Here's the drawing with two shaded views (mm, measured from the low corner). I have some questions. A direction names the side the tool comes from. Round coordinates to 2 decimals unless told otherwise and drop trailing zeros. Loops run counter-clockwise (first coordinate to the right, second up) from the corner with the lowest first, then second, coordinate; pieces in that order, holes last. Notation, with made-up numbers: (71, 35) -> (125, 35) arc R13 cw to (125, 39) -> close; hole circle Ø10 at (67, -32.75). An arc over 180 degrees is marked (long way). Write item = value, one per line.
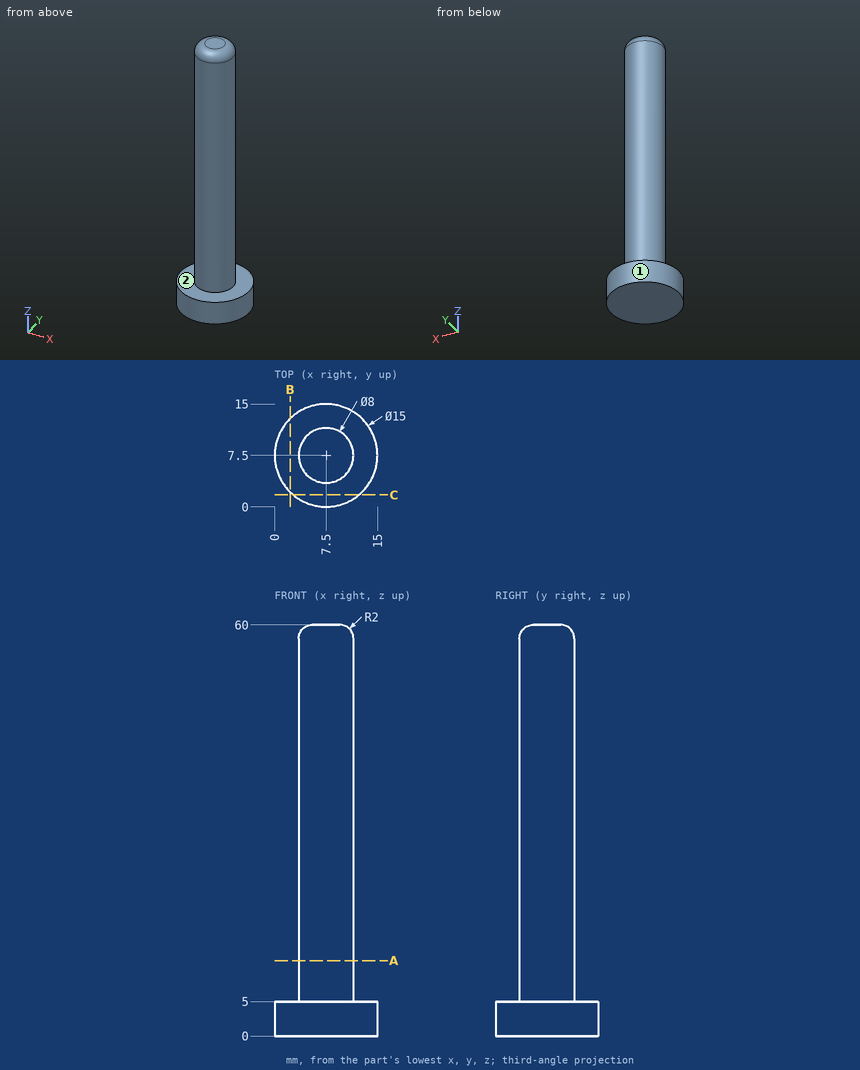
1. Suppose I cut it at A-A, the plane z = 11. List the corners of the cut face in (x, y) for me, and give its area (3 significant figures).
Entries:
outline = circle Ø8 at (7.5, 7.5)
area = 50.3 mm²
2. For the marked faces 1 and 2, which set-ups out of +Z, -Z, +X, -X, +Y, -Y let a thin tool reach every point of the face, with its end or its side?
Entries:
face_1 = +Z, -Z
face_2 = +Z
3. I need wall thicknesses on line 1 (Z direction, x = 11.75, y = 3.5); line 2 (X direction, y = 9.25, z = 34.5); line 3 (Y direction, x = 10.75, z = 42). Which ranges of each line are inside material? Lowest first, please. Write a range as [from, to].
Entries:
line_1 = [0, 5]
line_2 = [3.9, 11.1]
line_3 = [5.17, 9.83]
4. Suppose I cut it at B-B, the plane x = 2.25. List the corners of the cut face in (y, z) for me, and give its area (3 significant figures).
Entries:
outline = (2.14, 0) -> (12.86, 0) -> (12.86, 5) -> (2.14, 5) -> close
area = 53.6 mm²
5. I'm going to push flat-ended pins straight in: pin 1 (3 mm diameter, centred on x = 4, z = 11.5, fed in from -Y); pin 2 (5 mm diameter, centred on x = 5.5, z = 10, fed in from +Y); pin 3 (3 mm diameter, centred on y = 4.5, z = 42.5, fed in from -X). Where does each tip first touch, or does it pass through?
Entries:
pin_1 = 4.04
pin_2 = 11.5
pin_3 = 3.79
6. Suppose I cut it at C-C, the plane y = 1.75. List the corners of the cut face in (x, z) for me.
Entries:
outline = (2.68, 0) -> (12.32, 0) -> (12.32, 5) -> (2.68, 5) -> close
